from build123d import *

# Parameters (mm, degrees)
CROQUIS2_R              = 48
CROQUIS2_R_2            = 13.5
CROQUIS2_R_3            = 5.5
SALIENTE_EXTRUIR1_DEPTH = 10
CROQUIS4_R              = 48
CROQUIS4_R_2            = 13.5
CROQUIS4_R_3            = 5.5
SALIENTE_EXTRUIR2_DEPTH = 10
CROQUIS6_R              = 18
CROQUIS6_R_2            = 13.5
CROQUIS8_R              = 9
CORTAR_EXTRUIR1_DEPTH   = 3
CROQUIS9_R              = 9
CORTAR_EXTRUIR2_DEPTH   = 3


with BuildPart() as part:
    # Croquis2 → Saliente-Extruir1 (new body)
    with BuildSketch(Plane(origin=(0, 0, 0), x_dir=(0, 0, -1), z_dir=(1, 0, 0))):
        Circle(CROQUIS2_R)
        Circle(CROQUIS2_R_2, mode=Mode.SUBTRACT)
        with Locations((0, 33)):
            Circle(CROQUIS2_R_3, mode=Mode.SUBTRACT)
        with Locations((33, 0)):
            Circle(CROQUIS2_R_3, mode=Mode.SUBTRACT)
        with Locations((0, -33)):
            Circle(CROQUIS2_R_3, mode=Mode.SUBTRACT)
        with Locations((-33, 0)):
            Circle(CROQUIS2_R_3, mode=Mode.SUBTRACT)
    extrude(amount=SALIENTE_EXTRUIR1_DEPTH)



with BuildPart() as body_2:
    # Croquis4 → Saliente-Extruir2 (new body)
    with BuildSketch(Plane.XY.offset(150)):
        with Locations((150, 0)):
            Circle(CROQUIS4_R)
        with Locations((150, 0)):
            Circle(CROQUIS4_R_2, mode=Mode.SUBTRACT)
        with Locations((150, 33)):
            Circle(CROQUIS4_R_3, mode=Mode.SUBTRACT)
        with Locations((183, 0)):
            Circle(CROQUIS4_R_3, mode=Mode.SUBTRACT)
        with Locations((150, -33)):
            Circle(CROQUIS4_R_3, mode=Mode.SUBTRACT)
        with Locations((117, 0)):
            Circle(CROQUIS4_R_3, mode=Mode.SUBTRACT)
    extrude(amount=-SALIENTE_EXTRUIR2_DEPTH)


with BuildPart() as part_1:
    add(part.part)

    add(body_2.part)  # Barrer1 merges body 2
    # Barrer1: sweep along a path in Croquis5
    with BuildLine(Plane(origin=(0, 0, 0), x_dir=(1, 0, 0), z_dir=(0, 1, 0))) as barrer1_path:
        ThreePointArc((10, 0), (108.994949366, -41.005050634), (150, -140))
    # Croquis6 → Barrer1 (sweep)
    with BuildSketch(Plane(origin=(10, 0, 0), x_dir=(0, 0, -1), z_dir=(1, 0, 0))):
        Circle(CROQUIS6_R)
        Circle(CROQUIS6_R_2, mode=Mode.SUBTRACT)
    sweep(path=barrer1_path.line)

    # Croquis8 → Cortar-Extruir1 (cut)
    with BuildSketch(Plane(origin=(10, 0, 0), x_dir=(0, 0, -1), z_dir=(1, 0, 0))):
        with Locations((0, 33)):
            Circle(CROQUIS8_R)
        with Locations((33, 0)):
            Circle(CROQUIS8_R)
        with Locations((0, -33)):
            Circle(CROQUIS8_R)
        with Locations((-33, 0)):
            Circle(CROQUIS8_R)
    extrude(amount=-CORTAR_EXTRUIR1_DEPTH, mode=Mode.SUBTRACT)

    # Croquis9 → Cortar-Extruir2 (cut)
    with BuildSketch(Plane(origin=(0, 0, 140), x_dir=(-1, 0, 0), z_dir=(0, 0, -1))):
        with Locations((-150, 33)):
            Circle(CROQUIS9_R)
        with Locations((-117, 0)):
            Circle(CROQUIS9_R)
        with Locations((-150, -33)):
            Circle(CROQUIS9_R)
        with Locations((-183, 0)):
            Circle(CROQUIS9_R)
    extrude(amount=-CORTAR_EXTRUIR2_DEPTH, mode=Mode.SUBTRACT)


solid = part_1.part
Input: part model. Units: mm. Frame: model coordinates. A direction names the side the tool comes from. Round coordinates to 2 decimals unless told otherwise and drop trailing zeros. Loops run counter-clockwise (first coordinate to the right, second up) from the corner with the lowest first, then second, coordinate; pieces in that order, holes last. Notation, with made-up numbers: (34.5, 80.25) -> (58.5, 80.25) arc R35 cw to (58.5, 113.25) -> close; hole circle Ø1 at (-18, -39.75). An arc over 180 degrees is marked (long way). Answer as a JSON object with one key per item and string values. Group by question number.
1) Section query A-A on z = -33. Output: boundary loops of the cut face in (x, y), plus the area to 3 significant figures.
2) Draft query along Z for faces 1 (the flat face through (7, -37, 4)), 2 (the cylindrical face through (108.416, 2.703, 141.479)), 3 (the flat face through (187, -4, 143)), 4 (the cylindrical face through (177.505, 0.242, 146.549)). Return one class per face: +Z half, -Z half, draft (parallel to the pull), parting line (faces both ways), or undercut.
3) Pin query (flat end, axial travel): pin 1 (9 mm diameter, centred on y = -0.5, z = -34, fed in from +X); pin 2 (14.5 mm diameter, centred on x = 117, y = 0, fed in from -Z); pin 3 (3 mm diameter, centred on x = 24.5, z = 13.5, fed in from -Y); pin 4 (9 mm diameter, centred on x = 150, y = -33, fed in from -Z). Return the tip coordinate at first contact, or that it passes through.
4) Ray query, L1, parallel to Y at x = 7.9, z = 0; L2, parallel to Y at x = 150, z = 145; L3, parallel to X at y = 10.5, z = 41. Return the intervals inside material, ascending.
5) Reachability of faces 5 (the cylindrical face through (4.93, -13.18, 2.93)), 6 (the flat face through (171, 1, 140)), 7 (the flat face through (154, -37, 143)) from +Z, -Z, +X, -X, +Y, -Y: full face, straight path, thin tool, end or side. Return the list, or none.
6) Section query B-B on x = 183. Output: boundary loops of the cut face in (y, z), plus the area to 3 significant figures.
7) Section query C-C on y = 0. State how many separate pieces and enclosed holes the cut face has, plus the area to 3 significant figures.
Reply:
{
 "1": {"outline": "(0, -34.86) -> (10, -34.86) -> (10, -9) -> (7, -9) -> (7, -5.5) -> (0, -5.5) -> close; (0, 5.5) -> (7, 5.5) -> (7, 9) -> (10, 9) -> (10, 34.86) -> (0, 34.86) -> close", "area": "566 mm2"},
 "2": {"face 1": "undercut", "face 2": "undercut", "face 3": "-Z half", "face 4": "draft"},
 "3": {"pin 1": "stops at x = 7", "pin 2": "stops at z = 17.47", "pin 3": "stops at y = -14.11", "pin 4": "passes through"},
 "4": {"L1": "y = -48 to -42, -24 to -13.5, 13.5 to 24, 42 to 48", "L2": "y = -48 to -38.5, -27.5 to -13.5, 13.5 to 27.5, 38.5 to 48", "L3": "x = 0 to 10, 86.94 to 96.57, 120.67 to 128.77"},
 "5": {"face 5": "-X", "face 6": "none", "face 7": "-Z"},
 "6": {"outline": "(-34.86, 140) -> (-9, 140) -> (-9, 143) -> (-5.5, 143) -> (-5.5, 150) -> (-34.86, 150) -> close; (5.5, 143) -> (9, 143) -> (9, 140) -> (34.86, 140) -> (34.86, 150) -> (5.5, 150) -> close", "area": "566 mm2"},
 "7": {"separate pieces": "6", "enclosed holes": "0", "area": "2,840 mm2"}
}
